from build123d import *

# Parameters (mm, degrees)
SKETCH_1_R          = 4
EXTRUDE_1_DEPTH     = 8
SKETCH_2_W          = 5
SKETCH_2_H          = 5
EXTRUDE_2_DEPTH     = 5.2
SKETCH_3_R          = 2.5
EXTRUDE_3_DEPTH     = 2.8
SKETCH_4_OUTSIDE_W  = 15.306
SKETCH_4_OUTSIDE_H  = 15.306
SKETCH_4_OUTSIDE_R  = 2.25
CUT_EXTRUDE_1_DEPTH = 1.5
CHAMFER_1_SIZE      = 0.5


with BuildPart() as part:
    # 草图1 → 凸台-拉伸1 (new, symmetric)
    with BuildSketch(Plane.XY):
        Circle(SKETCH_1_R)
    extrude(amount=EXTRUDE_1_DEPTH, both=True)

    # 草图2 → 凸台-拉伸2 (add)
    with BuildSketch(Plane.XY.offset(8)):
        Rectangle(SKETCH_2_W, SKETCH_2_H)
    extrude(amount=EXTRUDE_2_DEPTH)

    # 草图3 → 凸台-拉伸3 (add)
    with BuildSketch(Plane.XY.offset(13.2)):
        Circle(SKETCH_3_R)
    extrude(amount=EXTRUDE_3_DEPTH)

    # 草图4 outside → 切除-拉伸1 (cut)
    with BuildSketch(Plane.XY.offset(13.2)):
        Rectangle(SKETCH_4_OUTSIDE_W, SKETCH_4_OUTSIDE_H)
        Circle(SKETCH_4_OUTSIDE_R, mode=Mode.SUBTRACT)
    extrude(amount=CUT_EXTRUDE_1_DEPTH, mode=Mode.SUBTRACT)

    # 倒角1
    chamfer_1_edges = [part.edges().sort_by_distance(p)[0] for p in [
        (-2.5, 0, 16),
    ]]
    chamfer(chamfer_1_edges, length=CHAMFER_1_SIZE)


solid = part.part
Can you work these out from the model? Positions are in its coordinate system, mm. A direction names the side the tool comes from. Coordinates: 2 decimals unless noted, no trailing zeros. Loops run counter-clockwise (first coordinate to the right, second up) from the corner with the lowest first, then second, coordinate; pieces in that order, holes last. Notation, with made-up numbers: M -37,-10.75 L 14,-10.75 A20 ccw 14,25.25 Z; hole C 61,67 d4. An arc over 180 degrees is marked long. Return JSON: item names as keys, results as strings. Group by question number.
Item 1: Thinking about a two-plate mould opening in Z: for faces 6 (the cylindrical face through (-0.29, 2.23, 13.94)), 7 (the cylindrical face through (-0.867, -3.905, 0.112)), 8 (the flat face through (0, 0, 16)), which applies, released by +Z, released by -Z, zero draft, split by the parting line, or undercut?
Item 2: If I drill on L1, parallel to Y at x = -1.75, z = 11; L2, parallel to Z at x = 3.25, y = -1.25, over which ranges is the centre line in solid material (lowest first)? Write a range as from..to.
Item 3: Imagine slicing it at C-C (z = -3). Please give me the cut outline in (x, y), and give its area (3 significant figures).
Item 4: On a 3-axis mill with a long thin cutter (end or side, diameter ignored), from which of +Z, -Z, +X, -X, +Y, -Y can I reach the whole of each face in a straight line? I mean faces 1 (the cylindrical face through (-0.54, -2.44, 15.09)), 2 (the flat face through (0, 2.5, 11)), 3 (the flat face through (-2, 2, 13.2)), 4 (the flat face through (2.5, 0, 11)), 5 (the flat face through (-2.5, 0, 11)). Say none if no direction works.
Item 5: Imagine slicing it at D-D (z = 8.25). Please give me the cut outline in (x, y).
Item 6: Imagine slicing it at A-A (y = 0). Please give me the cut outline in (x, z), and give its area (3 significant figures).
Item 7: I'm going to push flat-ended pins straight in: pin 1 Ø1.5 at (y, z) = (0.5, 9.5) entering from -X; pin 2 Ø4 at (x, z) = (0.5, 10.5) entering from +Y; pin 3 Ø2 at (y, z) = (3, 13.5) entering from +X. Where does each tip first touch, or does it pass through?
Verdict:
{
 "1": {"face 6": "undercut", "face 7": "zero draft", "face 8": "released by +Z"},
 "2": {"L1": "y = -2.5..2.5", "L2": "z = -8..8"},
 "3": {"outline": "C 0,0 d8", "area": "50.3 mm^2"},
 "4": {"face 1": "+Z", "face 2": "+Z, +X, -X, +Y", "face 3": "none", "face 4": "+Z, +X, +Y, -Y", "face 5": "+Z, -X, +Y, -Y"},
 "5": {"outline": "M -2.5,-2.5 L 2.5,-2.5 L 2.5,2.5 L -2.5,2.5 Z"},
 "6": {"outline": "M -4,-8 L 4,-8 L 4,8 L 2.5,8 L 2.5,13.2 L 2.25,13.2 L 2.25,14.7 L 2.5,14.7 L 2.5,15.5 L 2,16 L -2,16 L -2.5,15.5 L -2.5,14.7 L -2.25,14.7 L -2.25,13.2 L -2.5,13.2 L -2.5,8 L -4,8 Z", "area": "167 mm^2"},
 "7": {"pin 1": "stops at x = -2.5", "pin 2": "stops at y = 2.5", "pin 3": "stops at x = 2.5"}
}
